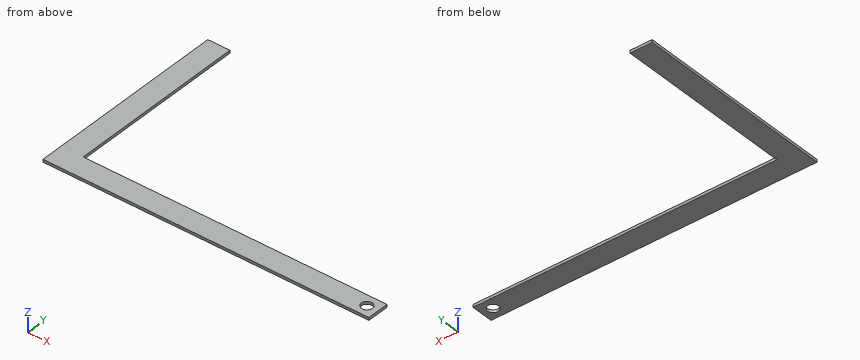
```python
from build123d import *

# Parameters (mm, degrees)
SKETCH1_W           = 374.65
SKETCH1_H           = 25.4
SKETCH1_R           = 6.35
BOSS_EXTRUDE1_DEPTH = 3.175
SKETCH2_W           = 25.4
SKETCH2_H           = 206.375
BOSS_EXTRUDE2_DEPTH = 3.175


with BuildPart() as part:
    # Sketch1 → Boss-Extrude1 (new body)
    with BuildSketch(Plane.XY):
        with Locations((187.325, 12.7)):
            Rectangle(SKETCH1_W, SKETCH1_H)
        with Locations((361.95, 12.7)):
            Circle(SKETCH1_R, mode=Mode.SUBTRACT)
    extrude(amount=BOSS_EXTRUDE1_DEPTH)

    # Sketch2 → Boss-Extrude2 (add)
    with BuildSketch(Plane.XY.offset(3.175)):
        with Locations((12.7, 128.5875)):
            Rectangle(SKETCH2_W, SKETCH2_H)
    extrude(amount=-BOSS_EXTRUDE2_DEPTH)


solid = part.part
```
Check sheet for the modelled part. Datum: model origin and axes. Units: mm. Coordinates: 2 decimals unless noted, no trailing zeros. Write each loop counter-clockwise with the first axis right and the second up, starting at its lowest first coordinate (ties: lowest second). Pieces come first, ordered by that corner, then holes. Notation, with made-up numbers: M -19,-3 L -2,-3 A25 cw -2,10 Z; hole C 20.25,-37 d11. An arc over 180 degrees is marked long. Write item = value, one per line. Start each with the question number.
1. Go/stop test with a flat-tipped pin: pin 1 (1 mm diameter, centred on x = 145.5, z = 2.5, fed in from +Y). Record where the tip stops, or that it passes through.
2. Sectioned sample at A-A (y = 12.7). Record the cut outline in (x, z) (3 decimals), then the cut area to 3 significant figures.
3. Sectioned sample at C-C (y = 112). Record the cut outline in (x, z) (3 decimals), then the cut area to 3 significant figures.
4. Sectioned sample at B-B (x = 361.95). Record the cut outline in (y, z) (3 decimals).
5. Thickness scan on probe 1 along Y at (x, z) = (361.95, 2.4); probe 2 along X at (y, z) = (152.5, 1.4). Record the ranges inside material, lowest first.
The answers:
q1.pin_1 = 25.4
q2.outline = M 0,0 L 355.6,0 L 355.6,3.175 L 0,3.175 Z; M 368.3,0 L 374.65,0 L 374.65,3.175 L 368.3,3.175 Z
q2.area = 1,150 mm²
q3.outline = M 0,0 L 25.4,0 L 25.4,3.175 L 0,3.175 Z
q3.area = 80.6 mm²
q4.outline = M 0,0 L 6.35,0 L 6.35,3.175 L 0,3.175 Z; M 19.05,0 L 25.4,0 L 25.4,3.175 L 19.05,3.175 Z
q5.probe_1 = 0 to 6.35, 19.05 to 25.4
q5.probe_2 = 0 to 25.4
